Design review of the part built by this model. Coordinates are the model's own, in mm. Face numbers are marked on the shaded views. A direction names the side the tool comes from. Coordinates: 2 decimals unless noted, no trailing zeros. Loops run counter-clockwise (first coordinate to the right, second up) from the corner with the lowest first, then second, coordinate; pieces in that order, holes last. Notation, with made-up numbers: M 80,-4 L 99,-4 A28 cw 99,29 Z; hole C -22.75,78.5 d5. An arc over 180 degrees is marked long. Answer as a JSON object with one key per item and string values. Group by question number.
1. Draft analysis for pull direction Y (two halves, no side actions). For the marked faces 6 and 7, state which applies: +Y half, -Y half, draft (parallel to the pull), parting line (faces both ways), or undercut.
2. To check wall thickness, follow probe 1 along Y at (x, z) = (2, -81); probe 2 along Y at (x, z) = (0, 76); probe 3 along Y at (x, z) = (14.5, 34). State the ranges of each line that lie inside material, in increasing order.
3. Insertion check: pin 1 (11 mm diameter, centred on x = 16, y = 280, fed in from +Z); pin 2 (4.5 mm diameter, centred on y = 19, z = -102.5, fed in from -X); pin 3 (12 mm diameter, centred on y = 82, z = -102, fed in from +X). Each pin has a flat end and moves straight along its axis. Give the tip position at first contact, or say it passes through.
4. Machinability: for the marked faces 1, 2, 3, 4 and 5, which of the approach directions +Z, -Z, +X, -X, +Y, -Y give a long, thin tool a straight path to every point of the face, cutting with its end or side? Answer none if there is none.
5. Consider section A-A (z = 3). State the section outline as (x, y) points, then the cut area to 3 significant figures.
6. Consider section C-C (y = -25). State the section outline as (x, z) points, then the cut area to 3 significant figures.
7. Consider section B-B (y = 55). State the section outline as (x, z) points.
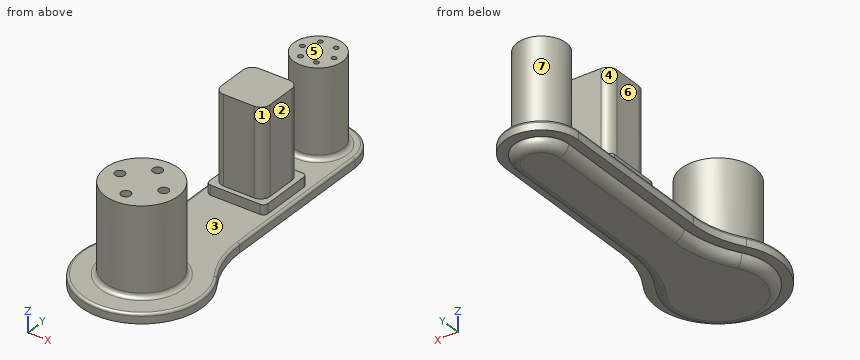
from build123d import *

# Parameters (mm, degrees)
SKETCH1_R             = 50
BOSS_EXTRUDE1_DEPTH   = 90
SKETCH1_R_2           = 75
BOSS_EXTRUDE1_2_DEPTH = 90
SKETCH2_R             = 10
SKETCH2_R_2           = 5
CUT_EXTRUDE1_DEPTH    = 40
BOSS_EXTRUDE2_DEPTH   = 20
BOSS_EXTRUDE3_DEPTH   = 20
FILLET1_R             = 19
SKETCH5_W             = 120
SKETCH5_H             = 120
BOSS_EXTRUDE4_DEPTH   = 20
SKETCH6_W             = 100
SKETCH6_H             = 100
BOSS_EXTRUDE5_DEPTH   = 180
FILLET2_R             = 19
FILLET3_R             = 9
FILLET4_R             = 5


with BuildPart() as part:
    # Sketch1 → Boss-Extrude1 (new, symmetric)
    with BuildSketch(Plane.XY):
        with Locations(Location((0, 250, 0), (0, 0, 180))):
            Circle(SKETCH1_R)
    extrude(amount=BOSS_EXTRUDE1_DEPTH, both=True)


with BuildPart() as body_2:
    # Sketch1 → Boss-Extrude1 2 (new, symmetric)
    with BuildSketch(Plane.XY):
        with Locations(Location((0, -250, 0), (0, 0, 180))):
            Circle(SKETCH1_R_2)
    extrude(amount=BOSS_EXTRUDE1_2_DEPTH, both=True)


with BuildPart() as cut_extrude1_tool:
    # Sketch2 → Cut-Extrude1 (new body)
    with BuildSketch(Plane.XY.offset(90)):
        with Locations((-45, -250)):
            Circle(SKETCH2_R)
        with Locations((0, -205)):
            Circle(SKETCH2_R)
        with Locations((45, -250)):
            Circle(SKETCH2_R)
        with Locations((0, -295)):
            Circle(SKETCH2_R)
        with Locations((-32.5, 250)):
            Circle(SKETCH2_R_2)
        with Locations((-16.25, 278.145825623)):
            Circle(SKETCH2_R_2)
        with Locations((16.25, 278.145825623)):
            Circle(SKETCH2_R_2)
        with Locations((32.5, 250)):
            Circle(SKETCH2_R_2)
        with Locations((16.25, 221.854174377)):
            Circle(SKETCH2_R_2)
        with Locations((-16.25, 221.854174377)):
            Circle(SKETCH2_R_2)
    extrude(amount=-CUT_EXTRUDE1_DEPTH)


with BuildPart() as part_1:
    add(part.part)

    # Cut-Extrude1: cut by cut_extrude1_tool
    add(cut_extrude1_tool.part, mode=Mode.SUBTRACT)



with BuildPart() as body_2_1:
    add(body_2.part)

    # Cut-Extrude1: cut by cut_extrude1_tool
    add(cut_extrude1_tool.part, mode=Mode.SUBTRACT)


with BuildPart() as part_2:
    add(part_1.part)

    add(body_2_1.part)  # Boss-Extrude2 merges body 2
    # Sketch3 → Boss-Extrude2 (add)
    with BuildSketch(Plane(origin=(0, 0, -90), x_dir=(-1, 0, 0), z_dir=(0, 0, -1))):
        with BuildLine():
            Line((-75, 250), (-75, -76.794919243))
            ThreePointArc((-75, -76.794919243), (-82.846215434, -132.264938866), (-105.769230769, -183.382661247))
            ThreePointArc((-105.769230769, -183.382661247), (0, -375), (105.769230769, -183.382661247))
            ThreePointArc((105.769230769, -183.382661247), (82.846215434, -132.264938866), (75, -76.794919243))
            Line((75, -76.794919243), (75, 250))
            ThreePointArc((75, 250), (0, 325), (-75, 250))
        make_face()
    extrude(amount=BOSS_EXTRUDE2_DEPTH)

    # Sketch4 → Boss-Extrude3 (add)
    with BuildSketch(Plane(origin=(0, 0, -110), x_dir=(-1, 0, 0), z_dir=(0, 0, -1))):
        with BuildLine():
            Line((-55, 250), (-55, -76.794919243))
            ThreePointArc((-55, -76.794919243), (-63.630836977, -137.811940828), (-88.846153846, -194.041435448))
            ThreePointArc((-88.846153846, -194.041435448), (0, -355), (88.846153846, -194.041435448))
            ThreePointArc((88.846153846, -194.041435448), (63.630836977, -137.811940828), (55, -76.794919243))
            Line((55, -76.794919243), (55, 250))
            ThreePointArc((55, 250), (0, 305), (-55, 250))
        make_face()
    extrude(amount=BOSS_EXTRUDE3_DEPTH)

    # Fillet1
    fillet1_edges = [part_2.edges().sort_by_distance(p)[0] for p in [
        (0, 305, -130),
        (55, 86.602540378, -130),
        (63.630836977, -137.811940828, -130),
        (0, -355, -130),
        (-63.630836977, -137.811940828, -130),
        (-55, 86.602540378, -130),
    ]]
    fillet(fillet1_edges, radius=FILLET1_R)

    # Sketch5 → Boss-Extrude4 (add)
    with BuildSketch(Plane.XY.offset(-90)):
        with Locations((0, 75)):
            Rectangle(SKETCH5_W, SKETCH5_H)
    extrude(amount=BOSS_EXTRUDE4_DEPTH)

    # Sketch6 → Boss-Extrude5 (add)
    with BuildSketch(Plane.XY.offset(-70)):
        with Locations((0, 75)):
            Rectangle(SKETCH6_W, SKETCH6_H)
    extrude(amount=BOSS_EXTRUDE5_DEPTH)

    # Fillet2
    fillet2_edges = [part_2.edges().sort_by_distance(p)[0] for p in [
        (-50, 25, 20),
        (50, 25, 20),
        (50, 125, 20),
        (-50, 125, 20),
    ]]
    fillet(fillet2_edges, radius=FILLET2_R)

    # Fillet3
    fillet3_edges = [part_2.edges().sort_by_distance(p)[0] for p in [
        (60, 15, -80),
        (60, 135, -80),
        (-60, 135, -80),
        (-60, 15, -80),
        (50, 250, -90),
        (75, -250, -90),
    ]]
    fillet(fillet3_edges, radius=FILLET3_R)

    # Fillet4
    fillet4_edges = [part_2.edges().sort_by_distance(p)[0] for p in [
        (0, 325, -90),
        (75, 86.602540378, -90),
        (82.846215434, -132.264938866, -90),
        (0, -375, -90),
        (-82.846215434, -132.264938866, -90),
        (-75, 86.602540378, -90),
    ]]
    fillet(fillet4_edges, radius=FILLET4_R)


solid = part_2.part
Findings below:
{
 "1": {"face 6": "draft", "face 7": "undercut"},
 "2": {"probe 1": "y = -324.97 to -175.03, 15 to 135, 200.04 to 299.96", "probe 2": "y = -325 to -305, -285 to -215, -195 to -175, 25 to 125, 200 to 300", "probe 3": "y = -323.58 to -176.42, 25 to 125, 202.15 to 297.85"},
 "3": {"pin 1": "stops at z = 90", "pin 2": "stops at x = -75", "pin 3": "stops at x = 75"},
 "4": {"face 1": "+Z, +X", "face 2": "+Z, +X, +Y", "face 3": "+Z", "face 4": "+Z, -X", "face 5": "+Z, +X, -X, +Y"},
 "5": {"outline": "C 0,-250 d150; M -50,44 A19 ccw -31,25 L 31,25 A19 ccw 50,44 L 50,106 A19 ccw 31,125 L -31,125 A19 ccw -50,106 Z; C 0,250 d100", "area": "35,200 mm^2"},
 "6": {"outline": "M -75,-110 L -55,-110 L -55,-111 A19 ccw -36,-130 L 36,-130 A19 ccw 55,-111 L 55,-110 L 75,-110 L 75,-95 A5 ccw 70,-90 L -70,-90 A5 ccw -75,-95 Z", "area": "5,030 mm^2"},
 "7": {"outline": "M -75,-110 L -55,-110 L -55,-111 A19 ccw -36,-130 L 36,-130 A19 ccw 55,-111 L 55,-110 L 75,-110 L 75,-95 A5 ccw 70,-90 L 60,-90 L 60,-70 L 50,-70 L 50,110 L -50,110 L -50,-70 L -60,-70 L -60,-90 L -70,-90 A5 ccw -75,-95 Z"}
}
